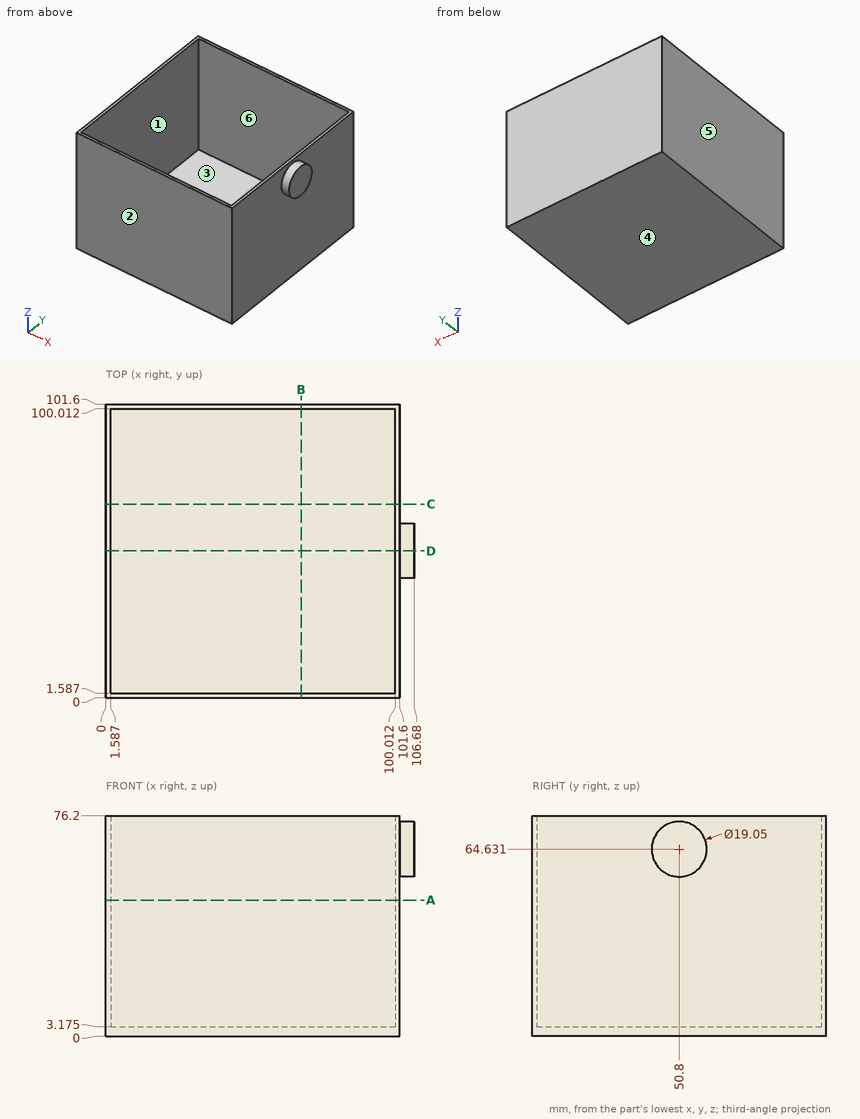
Design review of the part shown in the three views and the two pictorial views. Dimensions are in mm from the part's minimum x, y and z. A direction names the side the tool comes from. Coordinates: 2 decimals unless noted, no trailing zeros. Write each loop counter-clockwise with the first axis right and the second up, starting at its lowest first coordinate (ties: lowest second). Pieces come first, ordered by that corner, then holes. Notation, with made-up numbers: (23.5, 43) -> (56.5, 43) arc R25 cw to (56.5, 55) -> close; hole circle Ø11 at (34, 11). An arc over 180 degrees is marked (long way). Answer in a Markdown table with one row per item.
1. We need section D-D, the plane y = 50.8. State the section outline as (x, z) points (1 decimal).
Answers below:
| item | result |
|---|---|
| outline | (0, 0) -> (101.6, 0) -> (101.6, 55.1) -> (106.7, 55.1) -> (106.7, 74.2) -> (101.6, 74.2) -> (101.6, 76.2) -> (100, 76.2) -> (100, 3.2) -> (1.6, 3.2) -> (1.6, 76.2) -> (0, 76.2) -> close |
2. We need section A-A, the plane z = 47. State the section outline as (x, y) points.
Answers below:
| item | result |
|---|---|
| outline | (0, 0) -> (101.6, 0) -> (101.6, 101.6) -> (0, 101.6) -> close; hole (1.59, 1.59) -> (100.01, 1.59) -> (100.01, 100.01) -> (1.59, 100.01) -> close |
3. We need section B-B, the plane x = 67.5. State the section outline as (y, z) points (1 decimal).
Answers below:
| item | result |
|---|---|
| outline | (0, 0) -> (101.6, 0) -> (101.6, 76.2) -> (100, 76.2) -> (100, 3.2) -> (1.6, 3.2) -> (1.6, 76.2) -> (0, 76.2) -> close |
4. Clearance check with a flat-ended pin moving along its axis: pin 1 Ø4 at (x, y) = (18, 43) entering from +Z (1 decimal). State where the tip first meets the part, or that it passes through.
Answers below:
| item | result |
|---|---|
| pin 1 | stops at z = 3.2 |
5. Draft analysis for pull direction X (two halves, no side actions). For the marked faces 3, 4, 5 and 6, state which applies: +X half, -X half, draft (parallel to the pull), parting line (faces both ways), or undercut.
Answers below:
| item | result |
|---|---|
| face 3 | undercut |
| face 4 | draft |
| face 5 | -X half |
| face 6 | undercut |
6. Wall thickness on probe 1 along X at (y, z) = (97, 49); probe 2 along Z at (x, y) = (62, 24) (1 decimal): over which ranges is each line inside the solid? List them lowest first. Write a range as [from, to].
Answers below:
| item | result |
|---|---|
| probe 1 | x = [0, 1.59], [100.01, 101.6] |
| probe 2 | z = [0, 3.2] |
7. For the marked faces 1 and 2, list the 3-axis set-ups (+Z, -Z, +X, -X, +Y, -Y) from which the entire face can be reached by the end or side of a thin tool; tool diameter is ignored.
Answers below:
| item | result |
|---|---|
| face 1 | +Z |
| face 2 | +Z, -Z, +X, -X, -Y |
